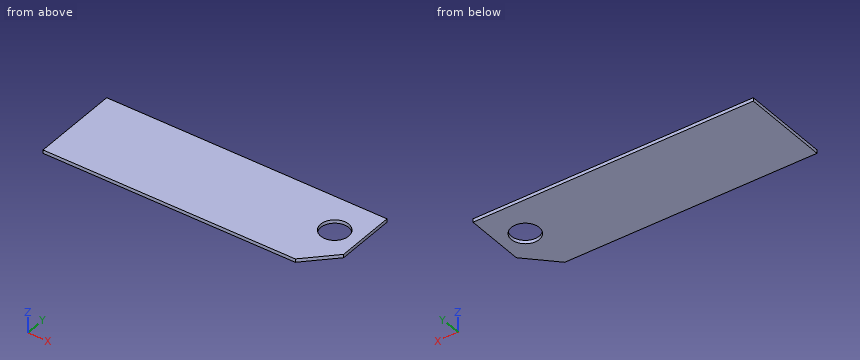
from build123d import *

# Parameters (mm, degrees)
SKETCH1_R           = 25
BOSS_EXTRUDE1_DEPTH = 6
SCALE1_SCALE        = 0.75


with BuildPart() as part:
    # Sketch1 → Boss-Extrude1 (new body)
    with BuildSketch(Plane.XY.offset(6)):
        Polygon((-200, -90), (250, -90), (300, -40), (300, 66.5), (-200, 66.5), align=None)
        with Locations((255, 0)):
            Circle(SKETCH1_R, mode=Mode.SUBTRACT)
    extrude(amount=-BOSS_EXTRUDE1_DEPTH)


with BuildPart() as part_1:
    # Scale1: scaled about (40.748726514, -11.031575069, 3)
    add(part.part.scale(SCALE1_SCALE).moved(Location((10.187181628, -2.757893767, 0.75))))


solid = part_1.part
Source: CAD feature listing. Evaluate the final solid. Frame: model axes, mm. Coordinates: 2 decimals unless noted, no trailing zeros. Loops run counter-clockwise (first coordinate to the right, second up) from the corner with the lowest first, then second, coordinate; pieces in that order, holes last. Notation, with made-up numbers: (-3.5, 64.25) - (1.5, 64.25) arc R21 cw to (1.5, 83.25) - close; hole circle Ø4 at (-18.5, 14.5). An arc over 180 degrees is marked (long way). One line per item, written item: value. Start each with the question number.
1. Section A-A (x = 193.5). Return the cut outline in (y, z).
2. Section B-B (z = 2.6). Return the cut outline in (x, y).
3. Ray query, L1, parallel to X at y = -9.5, z = 1.25; L2, parallel to X at y = -16, z = 4.8; L3, parallel to Y at x = 203, z = 3.25. Return the intervals inside material, ascending.
4. Section C-C (y = -43). Return the cut outline in (x, z).
Verdict:
1. outline: (-70.26, 0.75) - (-19.75, 0.75) - (-19.75, 5.25) - (-70.26, 5.25) - close; (14.23, 0.75) - (47.12, 0.75) - (47.12, 5.25) - (14.23, 5.25) - close
2. outline: (-139.81, -70.26) - (197.69, -70.26) - (235.19, -32.76) - (235.19, 47.12) - (-139.81, 47.12) - close; hole circle Ø37.5 at (201.44, -2.76)
3. L1: x = -139.81 to 183.94, 218.93 to 235.19
3. L2: x = -139.81 to 188.16, 214.71 to 235.19
3. L3: y = -64.95 to -21.44, 15.93 to 47.12
4. outline: (-139.81, 0.75) - (224.95, 0.75) - (224.95, 5.25) - (-139.81, 5.25) - close
